Geometry: final body of the model. Coordinates: model frame, mm. Face numbers are marked on the shaded views. A direction names the side the tool comes from. Round coordinates to 2 decimals unless told otherwise and drop trailing zeros. Order: outer loops, then holes, each group sorted by start corner. A loop starts at its lowest first (then second) coordinate and runs counter-clockwise, first axis right, second up. Notation, with made-up numbers: M 7.5,-39.5 L 30.5,-39.5 A29 ccw 30.5,-9.5 Z; hole C 28,-9 d7. An arc over 180 degrees is marked long. Return JSON: item names as keys, results as strings. Group by question number.
Q1. Mould query, pull axis Y, two halves, no side actions, for the marked faces 1, 2, 3 and 4. Classes: released by +Y, released by -Y, zero draft, split by the parting line, or undercut.
Q2. Cut plane C-C on z = 32. Output: boundary loops of the cut face in (x, y).
Q3. Ray query, probe 1 along Z at (x, y) = (31, -21); probe 2 along Z at (x, y) = (90.5, 28.5); probe 3 along Y at (x, z) = (87.5, 14). Return the intervals inside material, ascending.
Q4. Access query for the marked faces 5, 6 and 7. Directions: +Z, -Z, +X, -X, +Y, -Y. A direction counts if a zero-diameter tool reaches every point of the face in a straight line with its end or side. Return the directions, or none.
Q5. Contact query for flat-ended pins moving along their axis: pin 1 (1 mm diameter, centred on x = 70.5, y = 8, fed in from +Z); pin 2 (8 mm diameter, centred on x = 96, z = 30.5, fed in from -Y); pin 3 (1.6 mm diameter, centred on y = -1, z = 34, fed in from -X). Output: stop coordinate, or through.
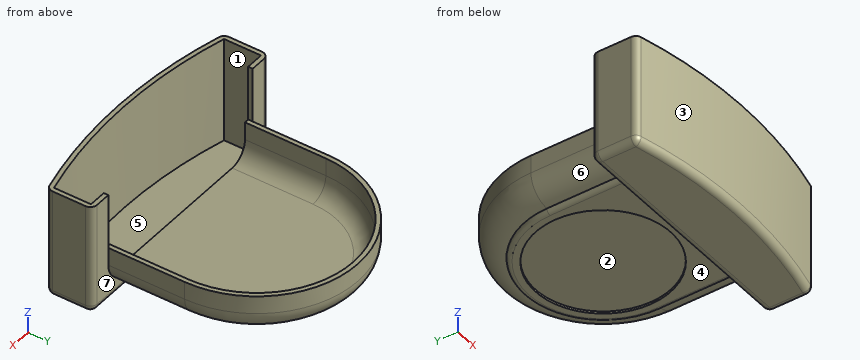
```python
from build123d import *

# Parameters (mm, degrees)
BOSS_EXTRUDE1_DEPTH = 49
CUT_EXTRUDE1_DEPTH  = 39
SHELL2_START        = 2
SHELL2_DEPTH        = 8
BOSS_EXTRUDE8_START = -81
SKETCH5_W           = 90
SKETCH5_H           = 18
BOSS_EXTRUDE8_DEPTH = 81
CUT_EXTRUDE2_DEPTH  = 142.941008873
FILLET1_R           = 10
SHELL4_DEPTH        = 34
SHELL4_2_ANGLE      = 180
CUT_EXTRUDE6_START  = -3
CUT_EXTRUDE6_DEPTH  = 3
BOSS_EXTRUDE9_DEPTH = 2
SKETCH10_R          = 30
CUT_EXTRUDE4_DEPTH  = 1
FILLET2_R           = 2
FILLET3_R           = 3


with BuildPart() as part:
    # Sketch1 → Boss-Extrude1 (new body)
    with BuildSketch(Plane.XY):
        with BuildLine():
            Line((0, 0), (110, 0))
            Line((110, 0), (110, -20))
            ThreePointArc((110, -20), (55, -27.200969375), (0, -20))
            Line((0, -20), (0, 0))
        make_face()
    extrude(amount=BOSS_EXTRUDE1_DEPTH)

    # Sketch3 → Cut-Extrude1 (cut)
    with BuildSketch(Plane.XY.offset(49)):
        with BuildLine():
            Line((10, 3.939932323), (10, -2))
            Line((10, -2), (2, -2))
            Line((2, -2), (2, -18.45731355))
            ThreePointArc((2, -18.45731355), (55, -25.200969375), (108, -18.45731355))
            Line((108, -18.45731355), (108, -2))
            Line((108, -2), (100, -2))
            Line((100, -2), (100, 3.939932323))
            Line((100, 3.939932323), (10, 3.939932323))
        make_face()
    extrude(amount=-CUT_EXTRUDE1_DEPTH, mode=Mode.SUBTRACT)

    # Shell2: read off the stored shape, not the designer's step
    # Shell2 outline → Shell2 (cut)
    with BuildSketch(Plane.XY.offset(SHELL2_START)):
        with BuildLine():
            Line((108, -18.45731355), (108, -2))
            Line((108, -2), (2, -2))
            Line((2, -2), (2, -18.45731355))
            ThreePointArc((2, -18.45731355), (55, -25.200969375), (108, -18.45731355))
        make_face()
    extrude(amount=SHELL2_DEPTH, mode=Mode.SUBTRACT)

    # Sketch5 → Boss-Extrude8 (add)
    with BuildSketch(Plane(origin=(0, 79, 0), x_dir=(1, 0, 0), z_dir=(0, 1, 0)).offset(BOSS_EXTRUDE8_START)):
        with Locations((55, -15.5)):
            Rectangle(SKETCH5_W, SKETCH5_H)
    extrude(amount=BOSS_EXTRUDE8_DEPTH)

    # Sketch6 → Cut-Extrude2 (cut, through all)
    with BuildSketch(Plane(origin=(0, 0, 6.5), x_dir=(-1, 0, 0), z_dir=(0, 0, -1))):
        with BuildLine():
            Line((-100, 84.89286518), (-10, 84.89286518))
            Line((-10, 84.89286518), (-10, 34))
            ThreePointArc((-10, 34), (-55, 79), (-100, 34))
            Line((-100, 34), (-100, 84.89286518))
        make_face()
    extrude(amount=-CUT_EXTRUDE2_DEPTH, mode=Mode.SUBTRACT)

    # Fillet1
    fillet1_edges = [part.edges().sort_by_distance(p)[0] for p in [
        (100, 17, 6.5),
        (10, 17, 6.5),
        (55, 79, 6.5),
    ]]
    fillet(fillet1_edges, radius=FILLET1_R)

    # Shell4: read off the stored shape, not the designer's step
    # Shell4 outline → Shell4 (cut)
    with BuildSketch(Plane(origin=(0, 0, 0), x_dir=(1, 0, 0), z_dir=(0, 1, 0))):
        with BuildLine():
            ThreePointArc((20, -8.5), (14.343145751, -10.843145751), (12, -16.5))
            Line((12, -16.5), (12, -24.5))
            Line((12, -24.5), (98, -24.5))
            Line((98, -24.5), (98, -16.5))
            ThreePointArc((98, -16.5), (95.656854249, -10.843145751), (90, -8.5))
            Line((90, -8.5), (20, -8.5))
        make_face()
    extrude(amount=SHELL4_DEPTH, mode=Mode.SUBTRACT)

    # Shell4 2 outline → Shell4 2 (revolve, cut)
    with BuildSketch(Plane(origin=(55, 34, 0), x_dir=(1, 0, 0), z_dir=(0, -1, 0))):
        with BuildLine():
            Line((0, 24.5), (0, 8.5))
            Line((0, 8.5), (35, 8.5))
            ThreePointArc((35, 8.5), (40.656854249, 10.843145751), (43, 16.5))
            Line((43, 16.5), (43, 24.5))
            Line((43, 24.5), (0, 24.5))
        make_face()
    revolve(axis=Axis((55, 34, 0), (0, 0, 1)), revolution_arc=SHELL4_2_ANGLE, mode=Mode.SUBTRACT)

    # Sketch12 → Cut-Extrude6 (cut)
    with BuildSketch(Plane(origin=(0, 0, 0), x_dir=(1, 0, 0), z_dir=(0, 1, 0)).offset(CUT_EXTRUDE6_START)):
        with BuildLine():
            Line((90, -8.5), (20, -8.5))
            ThreePointArc((20, -8.5), (14.343145751, -10.843145751), (12, -16.5))
            Line((12, -16.5), (12, -24.5))
            Line((12, -24.5), (98, -24.5))
            Line((98, -24.5), (98, -16.5))
            ThreePointArc((98, -16.5), (95.656854249, -10.843145751), (90, -8.5))
        make_face()
    extrude(amount=CUT_EXTRUDE6_DEPTH, mode=Mode.SUBTRACT)

    # Sketch9 → Boss-Extrude9 (add)
    with BuildSketch(Plane(origin=(0, 0, 6.5), x_dir=(-1, 0, 0), z_dir=(0, 0, -1))):
        with BuildLine():
            Line((-90, 0), (-20, 0))
            Line((-20, 0), (-20, 34))
            ThreePointArc((-20, 34), (-55, 69), (-90, 34))
            Line((-90, 34), (-90, 0))
        make_face()
    extrude(amount=BOSS_EXTRUDE9_DEPTH)

    # Sketch10 → Cut-Extrude4 (cut)
    with BuildSketch(Plane(origin=(0, 0, 4.5), x_dir=(-1, 0, 0), z_dir=(0, 0, -1))):
        with Locations((-55, 34)):
            Circle(SKETCH10_R)
    extrude(amount=-CUT_EXTRUDE4_DEPTH, mode=Mode.SUBTRACT)

    # Fillet2
    fillet2_edges = [part.edges().sort_by_distance(p)[0] for p in [
        (20, 17, 4.5),
        (55, 69, 4.5),
        (90, 17, 4.5),
    ]]
    fillet(fillet2_edges, radius=FILLET2_R - 0.0001)  # a hair under: the kernel refuses the full size

    # Fillet3
    fillet3_edges = [part.edges().sort_by_distance(p)[0] for p in [
        (55, 0, 0),
        (110, -10, 0),
        (55, -27.200969375, 0),
        (0, -10, 0),
        (0, 0, 24.5),
        (110, 0, 24.5),
        (110, -20, 24.5),
        (0, -20, 24.5),
    ]]
    fillet(fillet3_edges, radius=FILLET3_R)


solid = part.part
```
Result sheet:
{
 "1": {"face 1": "undercut", "face 2": "undercut", "face 3": "released by -Y", "face 4": "zero draft"},
 "2": {"outline": "M 0,-17.68 A3 ccw 2.26,-20.59 A213.64 ccw 107.74,-20.59 A3 ccw 110,-17.68 L 110,-3 A3 ccw 107,0 L 100,0 L 100,-2 L 108,-2 L 108,-18.46 A211.64 cw 2,-18.46 L 2,-2 L 10,-2 L 10,0 L 3,0 A3 ccw 0,-3 Z"},
 "3": {"probe 1": "z = 0 to 2", "probe 2": "z = 6.51 to 8.52", "probe 3": "y = -24.71 to -22.69, 61.54 to 64.66"},
 "4": {"face 5": "+Z", "face 6": "-Z, -X, +Y", "face 7": "-Z, +Y"},
 "5": {"pin 1": "stops at z = 8.5", "pin 2": "stops at y = -23.97", "pin 3": "stops at x = 0.25"}
}
